CAD build for the part. Positions are in the model's coordinates, mm. A direction names the side the tool comes from. Give positions to 0.01 mm unless a question says otherwise; leave off trailing zeros. Write each loop counter-clockwise with the first axis right and the second up, starting at its lowest first coordinate (ties: lowest second). Pieces come first, ordered by that corner, then holes. Notation, with made-up numbers: M 85.25,39 L 130.25,39 A20 cw 130.25,55 Z; hole C 68,89.25 d4. An arc over 180 degrees is marked long. One line per question, with ' | ' between items. Start each with the question number.
1. Flat gauge pin, fed straight in: pin 1 (2 mm diameter, centred on x = 1, y = 0, fed in from +Z). Where does the tip first touch, or does it go through?
2. Cut at D-D, the plane x = 3.75. Write the cut outline in (y, z), then the cut area to 3 significant figures.
3. Pull direction Y, two halves, no side cores. Call faces 4 (the face through (0, 2.426, 4)), 5 (the face through (-0.31, 1.39, 4.12)), 6 (the face through (0, 3.81, 5)), 7 (the face through (3, 0, 11.201)): released by +Y, released by -Y, zero draft, split by the parting line, or undercut.
4. Cut at B-B, the plane y = 0. Write the cut outline in (x, z).
5. Which spindle directions (+Z, -Z, +X, -X, +Y, -Y) get a long thin tool onto all of the face, cutting with end or side? Do faces 1 (the face through (6.414, 0, 4)), 2 (the face through (1.056, 0.105, 10.313)), 3 (the face through (0, 0, 0)). Say none if no direction does.
6. Cut at A-A, the plane z = 3.5. Write the cut outline in (x, y).
7. Wall check: L1, parallel to X at y = 0, z = 1.5; L2, parallel to Y at x = -1.5, z = 3.75; L3, parallel to X at y = 1.5, z = 5.25. Give the ranges that are in metal, low to high.
8. Cut at C-C, the plane x = 0. Write the cut outline in (y, z).
```python
from build123d import *

# Parameters (mm, degrees)
F0_W     = 15.621
F0_H     = 7.62
F1_DEPTH = 9.4488
F2_R     = 2.3876
F3_DEPTH = 1.7526
F4_W     = 12.827
F4_H     = 4.8514
F5_DEPTH = 8.128
F6_R     = 1.4224
F7_DEPTH = 8.128


with BuildPart() as f1:
    # F0 (on Top) → F1 (new body)
    with BuildSketch(Plane.XY):
        Rectangle(F0_W, F0_H)
    extrude(amount=F1_DEPTH)

    # F2 (on face) → F3 (join)
    with BuildSketch(Plane.XY.offset(9.4488)):
        with Locations((-3.4417, 0)):
            Circle(F2_R)
        with Locations((3.4417, 0)):
            Circle(F2_R)
    extrude(amount=F3_DEPTH)

    # F4 (on face) → F5 (cut)
    with BuildSketch(Plane(origin=(0, 0, 0), x_dir=(1, 0, 0), z_dir=(0, 0, -1))):
        Rectangle(F4_W, F4_H)
    extrude(amount=-F5_DEPTH, mode=Mode.SUBTRACT)

    # F6 (on face) → F7 (join)
    with BuildSketch(Plane(origin=(0, 0, 8.128), x_dir=(1, 0, 0), z_dir=(0, 0, -1))):
        Circle(F6_R)
    extrude(amount=F7_DEPTH)


solid = f1.part
```
Here are the results:
1) pin 1: z = 11.2
2) outline: M -3.81,0 L -2.43,0 L -2.43,8.13 L 2.43,8.13 L 2.43,0 L 3.81,0 L 3.81,9.45 L 2.37,9.45 L 2.37,11.2 L -2.37,11.2 L -2.37,9.45 L -3.81,9.45 Z | area: 40.9 mm^2
3) face 4: undercut | face 5: undercut | face 6: released by +Y | face 7: zero draft
4) outline: M -7.81,0 L -6.41,0 L -6.41,8.13 L -1.42,8.13 L -1.42,0 L 1.42,0 L 1.42,8.13 L 6.41,8.13 L 6.41,0 L 7.81,0 L 7.81,9.45 L 5.83,9.45 L 5.83,11.2 L 1.05,11.2 L 1.05,9.45 L -1.05,9.45 L -1.05,11.2 L -5.83,11.2 L -5.83,9.45 L -7.81,9.45 Z
5) face 1: -Z | face 2: +Z | face 3: -Z, +X, -X, +Y, -Y
6) outline: M -7.81,-3.81 L 7.81,-3.81 L 7.81,3.81 L -7.81,3.81 Z; C 0,0 d2.84; hole M -6.41,-2.43 L 6.41,-2.43 L 6.41,2.43 L -6.41,2.43 Z
7) L1: -7.81 to -6.41, -1.42 to 1.42, 6.41 to 7.81 | L2: -3.81 to -2.43, 2.43 to 3.81 | L3: -7.81 to -6.41, 6.41 to 7.81
8) outline: M -3.81,0 L -2.43,0 L -2.43,8.13 L -1.42,8.13 L -1.42,0 L 1.42,0 L 1.42,8.13 L 2.43,8.13 L 2.43,0 L 3.81,0 L 3.81,9.45 L -3.81,9.45 Z
